The model under review builds one solid part; all positions refer to its coordinate system, in mm. Face numbers are marked on the shaded views. A direction names the side the tool comes from. Round coordinates to 2 decimals unless told otherwise and drop trailing zeros. Loops run counter-clockwise (first coordinate to the right, second up) from the corner with the lowest first, then second, coordinate; pieces in that order, holes last. Notation, with made-up numbers: M 78.25,-24 L 82.25,-24 A13 cw 82.25,-6 Z; hole C -8.5,52.25 d4. An arc over 180 degrees is marked long. Return JSON: item names as keys, results as strings. Group by question number.
Q1. For the marked faces 1 and 2, list the 3-axis set-ups (+Z, -Z, +X, -X, +Y, -Y) from which the entire face can be reached by the end or side of a thin tool; tool diameter is ignored.
Q2. Consider section C-C (x = 30). State the section outline as (y, z) points (3 decimals).
Q3. To check wall thickness, follow line 1 along X through (y, z) = (17, -2); line 2 along Z through (x, y) = (43, 23); line 3 along Y through (x, z) = (-35, 27.5). State the ranges of each line that lie inside material, in increasing order.
Q4. Clearance check with flat-ended pins moving along their axes: pin 1 Ø6 at (x, y) = (-40, 40) entering from +Z; pin 2 Ø12.5 at (x, y) = (40, 40) entering from +Z; pin 3 Ø2 at (x, z) = (4, 28) entering from -Y. State where each tip first meets the part, or that it passes through.
Q5. Consider section B-B (x = -3). State the section outline as (y, z) points (3 decimals), and give its area (3 significant figures).
Q6. Consider section A-A (y = 17.5). State the section outline as (x, z) points.
Q7. Consider section D-D (y = -40). State the section outline as (x, z) points.
from build123d import *

# Parameters (mm, degrees)
CROQUIS1_W                       = 120
CROQUIS1_H                       = 120
CROQUIS1_R                       = 9.5
BRIDA_BASE1_DEPTH                = 3.03784
BRIDA_DE_ARISTA1_STRIP_W         = 18.50136
BRIDA_DE_ARISTA1_STRIP_H         = 3.03784
BRIDA_DE_ARISTA1_STRIP_CUT_DEPTH = 120
BRIDA_DE_ARISTA1_DEPTH           = 120
CORTAR_EXTRUIR1_REACH            = 161.883
CROQUIS9_R                       = 4.1
CORTAR_EXTRUIR2_REACH            = 125.693
CROQUIS10_R                      = 3.828194302
CROQUIS10_R_2                    = 3.588932158
CROQUIS10_R_3                    = 3.349670014


# Sheet-metal steps are written as plain solids
with BuildPart() as part:
    # Croquis1 → Brida base1 (new body)
    with BuildSketch(Plane.XY):
        Rectangle(CROQUIS1_W, CROQUIS1_H)
        with Locations((0, -35)):
            Circle(CROQUIS1_R, mode=Mode.SUBTRACT)
        with Locations((-30.310889132, 17.5)):
            Circle(CROQUIS1_R, mode=Mode.SUBTRACT)
        with Locations((30.310889132, 17.5)):
            Circle(CROQUIS1_R, mode=Mode.SUBTRACT)
    extrude(amount=-BRIDA_BASE1_DEPTH)

    # Brida de arista1 strip (across the edge) → Brida de arista1 strip cut (cut)
    with BuildSketch(Plane(origin=(60, 60, 0), x_dir=(0, -1, 0), z_dir=(-1, 0, 0))):
        with Locations((-3.03784, -1.51892)):
            Rectangle(BRIDA_DE_ARISTA1_STRIP_W, BRIDA_DE_ARISTA1_STRIP_H)
    extrude(amount=BRIDA_DE_ARISTA1_STRIP_CUT_DEPTH, mode=Mode.SUBTRACT)

    # Brida de arista1 section (across the edge) → Brida de arista1 (add)
    with BuildSketch(Plane(origin=(60, 60, 0), x_dir=(0, -1, 0), z_dir=(-1, 0, 0))):
        with BuildLine():
            Line((0, 3.175), (0, 86.96216))
            Line((0, 86.96216), (3.03784, 86.96216))
            Line((3.03784, 86.96216), (3.03784, 3.175))
            ThreePointArc((3.03784, 3.175), (3.96777597, 0.92993597), (6.21284, 0))
            Line((6.21284, 0), (6.21284, -3.03784))
            ThreePointArc((6.21284, -3.03784), (1.819698706, -1.218141294), (0, 3.175))
        make_face()
    extrude(amount=BRIDA_DE_ARISTA1_DEPTH)

    # Croquis9 → Cortar-Extruir1 (cut, up to next)
    with BuildSketch(Plane(origin=(0, 60, 0), x_dir=(1, 0, 0), z_dir=(0, 1, 0)), mode=Mode.PRIVATE) as cortar_extruir1_sk1:
        with Locations(Location((-30, -76.96216, 0), (0, 0, 270))):
            Circle(CROQUIS9_R)
    cortar_extruir1_tool1 = extrude(cortar_extruir1_sk1.sketch, amount=-CORTAR_EXTRUIR1_REACH, mode=Mode.PRIVATE) & part.part
    # Croquis9 → Cortar-Extruir1 (cut, up to next)
    with BuildSketch(Plane(origin=(0, 60, 0), x_dir=(1, 0, 0), z_dir=(0, 1, 0)), mode=Mode.PRIVATE) as cortar_extruir1_sk2:
        with Locations(Location((-30, -36.96216, 0), (0, 0, 270))):
            Circle(CROQUIS9_R)
    cortar_extruir1_tool2 = extrude(cortar_extruir1_sk2.sketch, amount=-CORTAR_EXTRUIR1_REACH, mode=Mode.PRIVATE) & part.part
    # Croquis9 → Cortar-Extruir1 (cut, up to next)
    with BuildSketch(Plane(origin=(0, 60, 0), x_dir=(1, 0, 0), z_dir=(0, 1, 0)), mode=Mode.PRIVATE) as cortar_extruir1_sk3:
        with Locations(Location((30, -36.96216, 0), (0, 0, 270))):
            Circle(CROQUIS9_R)
    cortar_extruir1_tool3 = extrude(cortar_extruir1_sk3.sketch, amount=-CORTAR_EXTRUIR1_REACH, mode=Mode.PRIVATE) & part.part
    # Croquis9 → Cortar-Extruir1 (cut, up to next)
    with BuildSketch(Plane(origin=(0, 60, 0), x_dir=(1, 0, 0), z_dir=(0, 1, 0)), mode=Mode.PRIVATE) as cortar_extruir1_sk4:
        with Locations(Location((30, -76.96216, 0), (0, 0, 270))):
            Circle(CROQUIS9_R)
    cortar_extruir1_tool4 = extrude(cortar_extruir1_sk4.sketch, amount=-CORTAR_EXTRUIR1_REACH, mode=Mode.PRIVATE) & part.part
    add(cortar_extruir1_tool1.solids().sort_by_distance((-30, 60, 76.96216))[0], mode=Mode.SUBTRACT)
    add(cortar_extruir1_tool2.solids().sort_by_distance((-30, 60, 36.96216))[0], mode=Mode.SUBTRACT)
    add(cortar_extruir1_tool3.solids().sort_by_distance((30, 60, 36.96216))[0], mode=Mode.SUBTRACT)
    add(cortar_extruir1_tool4.solids().sort_by_distance((30, 60, 76.96216))[0], mode=Mode.SUBTRACT)

    # Croquis10 → Cortar-Extruir2 (cut, up to next)
    with BuildSketch(Plane(origin=(0, 0, -3.03784), x_dir=(-1, 0, 0), z_dir=(0, 0, -1)), mode=Mode.PRIVATE) as cortar_extruir2_sk1:
        with Locations((40, 40)):
            Circle(CROQUIS10_R)
    cortar_extruir2_tool1 = extrude(cortar_extruir2_sk1.sketch, amount=-CORTAR_EXTRUIR2_REACH, mode=Mode.PRIVATE) & part.part
    # Croquis10 → Cortar-Extruir2 (cut, up to next)
    with BuildSketch(Plane(origin=(0, 0, -3.03784), x_dir=(-1, 0, 0), z_dir=(0, 0, -1)), mode=Mode.PRIVATE) as cortar_extruir2_sk2:
        with Locations((40, -40)):
            Circle(CROQUIS10_R_2)
    cortar_extruir2_tool2 = extrude(cortar_extruir2_sk2.sketch, amount=-CORTAR_EXTRUIR2_REACH, mode=Mode.PRIVATE) & part.part
    # Croquis10 → Cortar-Extruir2 (cut, up to next)
    with BuildSketch(Plane(origin=(0, 0, -3.03784), x_dir=(-1, 0, 0), z_dir=(0, 0, -1)), mode=Mode.PRIVATE) as cortar_extruir2_sk3:
        with Locations((-40, -40)):
            Circle(CROQUIS10_R_3)
    cortar_extruir2_tool3 = extrude(cortar_extruir2_sk3.sketch, amount=-CORTAR_EXTRUIR2_REACH, mode=Mode.PRIVATE) & part.part
    # Croquis10 → Cortar-Extruir2 (cut, up to next)
    with BuildSketch(Plane(origin=(0, 0, -3.03784), x_dir=(-1, 0, 0), z_dir=(0, 0, -1)), mode=Mode.PRIVATE) as cortar_extruir2_sk4:
        with Locations((-40, 40)):
            Circle(CROQUIS10_R)
    cortar_extruir2_tool4 = extrude(cortar_extruir2_sk4.sketch, amount=-CORTAR_EXTRUIR2_REACH, mode=Mode.PRIVATE) & part.part
    add(cortar_extruir2_tool1.solids().sort_by_distance((-40, 40, -3.03784))[0], mode=Mode.SUBTRACT)
    add(cortar_extruir2_tool2.solids().sort_by_distance((-40, -40, -3.03784))[0], mode=Mode.SUBTRACT)
    add(cortar_extruir2_tool3.solids().sort_by_distance((40, -40, -3.03784))[0], mode=Mode.SUBTRACT)
    add(cortar_extruir2_tool4.solids().sort_by_distance((40, 40, -3.03784))[0], mode=Mode.SUBTRACT)


solid = part.part
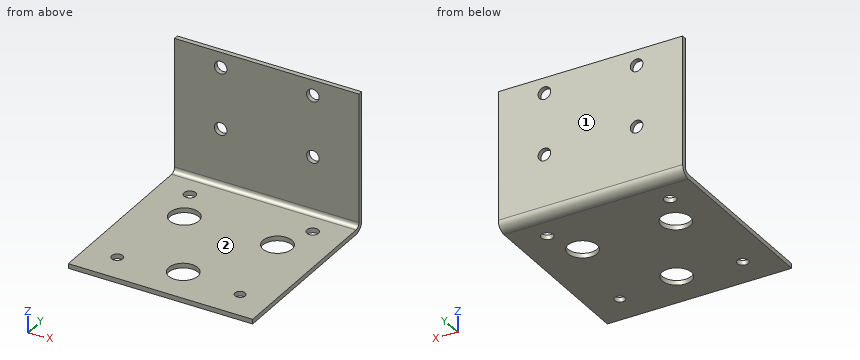
Values:
{
 "1": {"face 1": "+Z, -Z, +X, -X, +Y", "face 2": "+Z, +X, -X, -Y"},
 "2": {"outline": "M -60,-3.038 L 8.005,-3.038 L 8.005,0 L -60,0 Z; M 26.995,-3.038 L 53.787,-3.038 A6.213 ccw 60,3.175 L 60,32.862 L 56.962,32.862 L 56.962,3.175 A3.175 cw 53.787,0 L 26.995,0 Z; M 56.962,41.062 L 60,41.062 L 60,72.862 L 56.962,72.862 Z; M 56.962,81.062 L 60,81.062 L 60,86.962 L 56.962,86.962 Z"},
 "3": {"line 1": "x = -60 to -39.8, -20.82 to 20.82, 39.8 to 60", "line 2": "z = -3.04 to 0", "line 3": "y = 56.96 to 60"},
 "4": {"pin 1": "passes through", "pin 2": "stops at z = 0", "pin 3": "stops at y = 56.96"},
 "5": {"outline": "M -60,-3.038 L -44.014,-3.038 L -44.014,0 L -60,0 Z; M -25.986,-3.038 L 53.787,-3.038 A6.213 ccw 60,3.175 L 60,86.962 L 56.962,86.962 L 56.962,3.175 A3.175 cw 53.787,0 L -25.986,0 Z", "area": "568 mm2"},
 "6": {"outline": "M -60,-3.04 L -39.81,-3.04 L -39.81,0 L -60,0 Z; M -20.81,-3.04 L 20.81,-3.04 L 20.81,0 L -20.81,0 Z; M 39.81,-3.04 L 60,-3.04 L 60,0 L 39.81,0 Z"},
 "7": {"outline": "M -60,-3.04 L -43.59,-3.04 L -43.59,0 L -60,0 Z; M -36.41,-3.04 L -8.08,-3.04 L -8.08,0 L -36.41,0 Z; M 8.08,-3.04 L 36.65,-3.04 L 36.65,0 L 8.08,0 Z; M 43.35,-3.04 L 60,-3.04 L 60,0 L 43.35,0 Z"}
}
